```python
from build123d import *

# Parameters (mm, degrees)
EXTRUDE1_DEPTH          = 5
SKETCH2_OUTSIDE_W       = 36
SKETCH2_OUTSIDE_H       = 37.548
SKETCH2_OUTSIDE_R       = 5
CUT_EXTRUDE1_DEPTH      = 6
CUT_EXTRUDE1_TAPER      = 60
SKETCH4_R               = 3
CUT_EXTRUDE3_DEPTH      = 6
SKETCH12_OUTSIDE_W      = 15.214
SKETCH12_OUTSIDE_H      = 16.762
SKETCH12_OUTSIDE_R      = 3.6
CUT_EXTRUDE10_DEPTH     = 1.125
SKETCH15_W              = 0.381
SKETCH15_H              = 5.773502692
CUT_EXTRUDE_THIN2_DEPTH = 0.617
CIRPATTERN1_COUNT       = 6
SKETCH3_OUTSIDE_W       = 32.102
SKETCH3_OUTSIDE_H       = 33.65
SKETCH3_OUTSIDE_R       = 5
CUT_EXTRUDE2_DEPTH      = 4.875
CUT_EXTRUDE2_TAPER      = 60


with BuildPart() as part:
    # Sketch1 → Extrude1 (new body)
    with BuildSketch(Plane.XY):
        Polygon((0, 5.773502692), (-5, 2.886751346), (-5, -2.886751346), (0, -5.773502692), (5, -2.886751346), (5, 2.886751346), align=None)
    extrude(amount=-EXTRUDE1_DEPTH)

    # Sketch2 outside → Cut-Extrude1 (cut, through all)
    with BuildSketch(Plane.XY):
        Rectangle(SKETCH2_OUTSIDE_W, SKETCH2_OUTSIDE_H)
        Circle(SKETCH2_OUTSIDE_R, mode=Mode.SUBTRACT)
    extrude(amount=-CUT_EXTRUDE1_DEPTH, taper=CUT_EXTRUDE1_TAPER, mode=Mode.SUBTRACT)

    # Sketch4 → Cut-Extrude3 (cut, through all)
    with BuildSketch(Plane.XY):
        Circle(SKETCH4_R)
    extrude(amount=-CUT_EXTRUDE3_DEPTH, mode=Mode.SUBTRACT)

    # Sketch12 outside → Cut-Extrude10 (cut)
    with BuildSketch(Plane(origin=(0, 0, -5), x_dir=(-1, 0, 0), z_dir=(0, 0, -1))):
        Rectangle(SKETCH12_OUTSIDE_W, SKETCH12_OUTSIDE_H)
        Circle(SKETCH12_OUTSIDE_R, mode=Mode.SUBTRACT)
    extrude(amount=-CUT_EXTRUDE10_DEPTH, mode=Mode.SUBTRACT)

    # Sketch15 → Cut-Extrude-Thin2 (cut)
    with BuildSketch(Plane(origin=(0, 0, -5), x_dir=(-1, 0, 0), z_dir=(0, 0, -1))):
        with Locations((0, -2.886751346)):
            Rectangle(SKETCH15_W, SKETCH15_H)
    cut_extrude_thin2 = extrude(amount=-CUT_EXTRUDE_THIN2_DEPTH, mode=Mode.SUBTRACT)

    # CirPattern1: Cut-Extrude-Thin2 ×6 about axis
    cirpattern1_axis = Axis((0, 0, 0), (0, 0, 1))
    for i in range(1, CIRPATTERN1_COUNT):
        add(cut_extrude_thin2.rotate(cirpattern1_axis, i * 360 / CIRPATTERN1_COUNT), mode=Mode.SUBTRACT)

    # Sketch3 outside → Cut-Extrude2 (cut, through all)
    with BuildSketch(Plane(origin=(0, 0, -3.875), x_dir=(-1, 0, 0), z_dir=(0, 0, -1))):
        Rectangle(SKETCH3_OUTSIDE_W, SKETCH3_OUTSIDE_H)
        Circle(SKETCH3_OUTSIDE_R, mode=Mode.SUBTRACT)
    extrude(amount=-CUT_EXTRUDE2_DEPTH, taper=CUT_EXTRUDE2_TAPER, mode=Mode.SUBTRACT)


solid = part.part
```
The listing builds one solid part. Answer for the finished solid, in the listing's coordinates (mm). A direction names the side the tool comes from. Give positions to 0.01 mm unless a question says otherwise; leave off trailing zeros. Order: outer loops, then holes, each group sorted by start corner. A loop starts at its lowest first (then second) coordinate and runs counter-clockwise, first axis right, second up. Notation, with made-up numbers: M 28,-4.75 L 71,-4.75 A18 ccw 71,2.25 Z; hole C -36.75,76 d2. An arc over 180 degrees is marked long. Put each result on its own line as item: value. Start each with the question number.
Item 1: Which of the six approach directions +Z, -Z, +X, -X, +Y, -Y give full straight-line access (tool end or side, diameter ignored) to faces 1 (the face through (4.499, 2.583, -3.766)), 2 (the face through (-3.3, -2.2, -3.875))?
Item 2: Find the intervals of material crossed by line 1 along X through (y, z) = (-2.5, -0.6); line 2 along X through (y, z) = (0, -2.5); line 3 along Y through (x, z) = (2.5, -2.95), in increasing order.
Item 3: Flat-ended cylindrical pins translate along their axes: P1, Ø5, axis at x = -1.5, y = 1, coming from the -Z side; P2, Ø2, axis at x = -2, z = -3.5, coming from the -Y side; P3, Ø1, axis at y = 3.5, z = -1.5, coming from the -X side; P4, Ø0.5, axis at y = 3, z = -4.5, coming from the +X side. Find the tip coordinate at first contact, or state that the pin passes through.
Item 4: The part is cut by section A-A, the plane z = -0.9. Determine the outline of the cut face in (x, y), and give its area (3 significant figures).
Answer key:
1. face 1: -Z, +X, +Y
1. face 2: -Z
2. line 1: x = -5 to -1.66, 1.66 to 5
2. line 2: x = -5 to -3, 3 to 5
2. line 3: y = -4.33 to -1.66, 1.66 to 4.33
3. P1: stops at z = -5
3. P2: stops at y = -5.2
3. P3: stops at x = -4.8
3. P4: stops at x = 2.32
4. outline: M -5,-2.89 L 0,-5.77 L 5,-2.89 L 5,2.89 L 0,5.77 L -5,2.89 Z; hole C 0,0 d6
4. area: 58.3 mm²
